Source: three-view drawing plus pictorial views. Frame: mm from the lowest corner of the part. Give positions to 0.01 mm unless a question says otherwise; leave off trailing zeros. Write each loop counter-clockwise with the first axis right and the second up, starting at its lowest first coordinate (ties: lowest second). Pieces come first, ordered by that corner, then holes.
Q1. Pin query (flat end, axial travel): pin 1 (1 mm diameter, centred on y = 8, z = 28.5, fed in from +X); pin 2 (0.6 mm diameter, centred on x = 20, y = 16, fed in from +Z); pin 3 (1.5 mm diameter, centred on y = 2.5, z = 14, fed in from -X). Return the tip coordinate at first contact, or that it passes through.
Q2. Cut plane B-B on z = 10.5. Return the cut outline in (x, y).
Q3. Cut plane A-A on y = 2. Return the cut outline in (x, z).
Q4. Line query: L1, parallel to Y at x = 11.5, z = 38.8; L2, parallel to X at y = 17, z = 37 (1 decimal); L3, parallel to X at y = 11.25, z = 11. Output: solid intervals per line, ascending.
Q5. Cut plane D-D on y = 16.25. Return the cut outline in (x, z), plus the area to 3 significant figures.
Q6. Cut plane C-C on x = 5.75. Return the cut outline in (y, z).
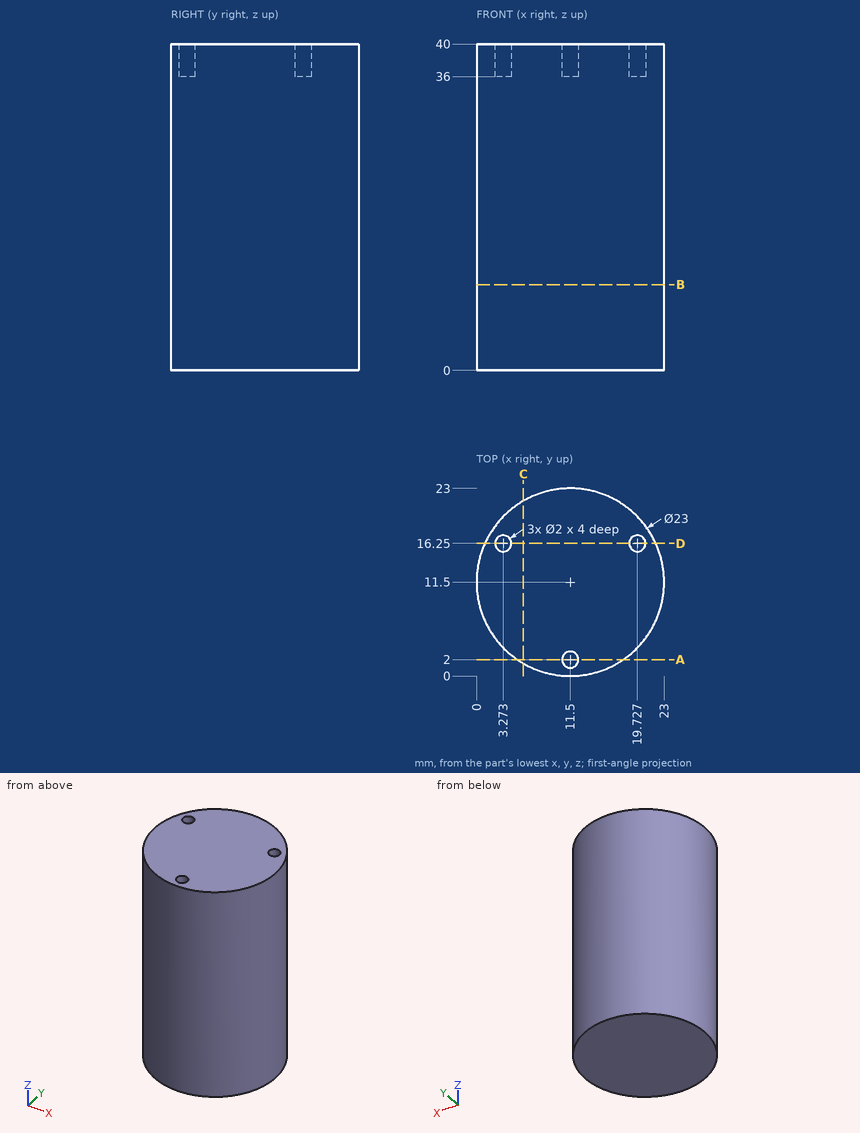
Data:
1. pin 1: stops at x = 22.6
1. pin 2: stops at z = 36
1. pin 3: stops at x = 3.49
2. outline: circle Ø23 at (11.5, 11.5)
3. outline: (5.02, 0) - (17.98, 0) - (17.98, 40) - (12.5, 40) - (12.5, 36) - (10.5, 36) - (10.5, 40) - (5.02, 40) - close
4. L1: y = 0 to 1, 3 to 23
4. L2: x = 1.4 to 2.6, 3.9 to 19.1, 20.4 to 21.6
4. L3: x = 0 to 23
5. outline: (1.03, 0) - (21.97, 0) - (21.97, 40) - (20.73, 40) - (20.73, 36) - (18.73, 36) - (18.73, 40) - (4.27, 40) - (4.27, 36) - (2.27, 36) - (2.27, 40) - (1.03, 40) - close
5. area: 822 mm2
6. outline: (1.54, 0) - (21.46, 0) - (21.46, 40) - (1.54, 40) - close
